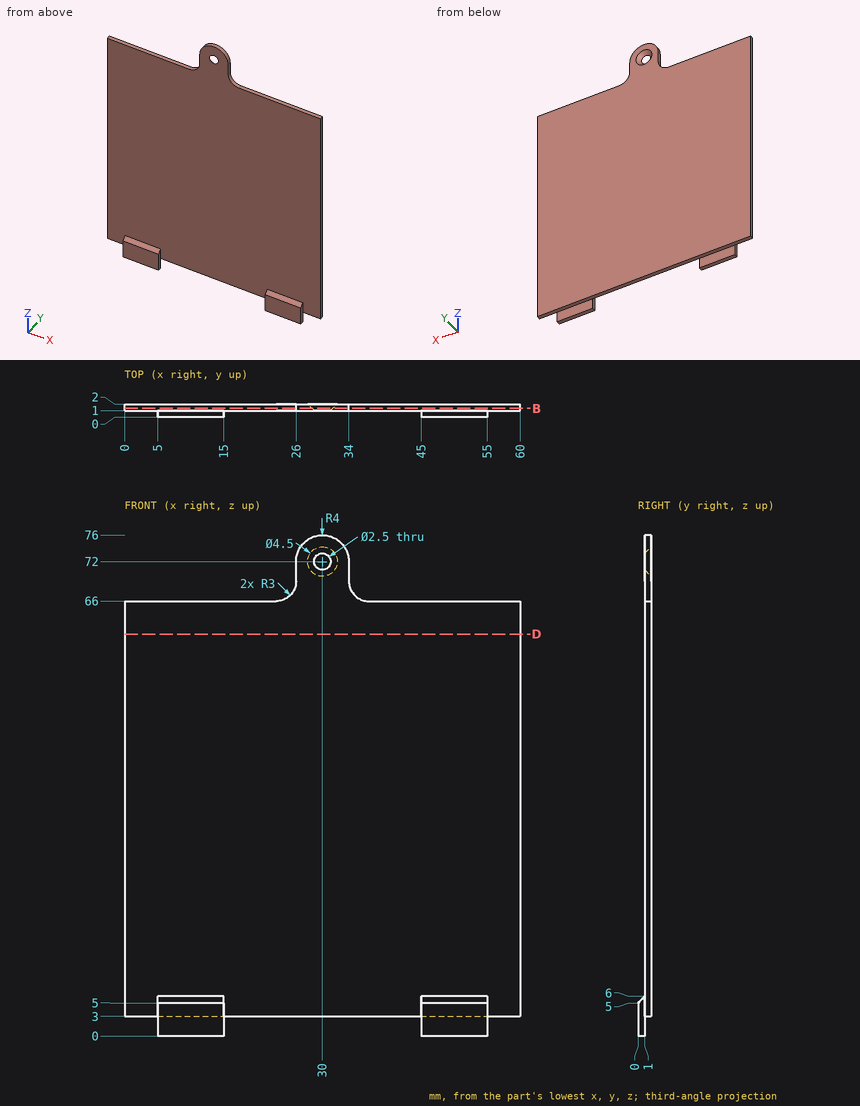
Drawing for the job (mm, zero at the part's lowest x, y, z). Give positions to 0.01 mm unless a question says otherwise; leave off trailing zeros. Order: outer loops, then holes, each group sorted by start corner. A loop starts at its lowest first (then second) coordinate and runs counter-clockwise, first axis right, second up. Notation, with made-up numbers: M 44.5,8 L 72.5,8 A21 cw 72.5,31 Z; hole C 23,15 d2. An arc over 180 degrees is marked long. Put each result on its own line as item: value. Start each with the question number.
(1) Saw through at D-D, the plane z = 61. Write the cut outline in (x, y).
(2) Saw through at B-B, the plane y = 1.35. Write the cut outline in (x, z), then the cut area to 3 significant figures.
(3) Flat gauge pins, fed straight in: pin 1 Ø0.5 at (y, z) = (0.5, 3.5) entering from +X; pin 2 Ø0.8 at (y, z) = (0.5, 2.5) entering from -X; pin 3 Ø3 at (x, z) = (15.5, 37.5) entering from -Y. Where does each tip first touch, or does it go through?
(4) Drill centre lines: line 1 along Z through (x, y) = (39, 1.5); line 2 along Y through (x, z) = (40.5, 39); line 3 along X through (y, z) = (1.05, 72). Where is each one in solid material? Low to high.
Check result:
1. outline: M 0,1 L 60,1 L 60,2 L 0,2 Z
2. outline: M 0,3 L 60,3 L 60,66 L 37,66 A3 cw 34,69 L 34,72 A4 ccw 26,72 L 26,69 A3 cw 23,66 L 0,66 Z; hole C 30,72 d3.2
2. area: 3,850 mm2
3. pin 1: stops at x = 55
3. pin 2: stops at x = 5
3. pin 3: stops at y = 1
4. line 1: z = 3 to 66
4. line 2: y = 1 to 2
4. line 3: x = 26 to 28.7, 31.3 to 34
